Autodesk Inventor part; units mm, degrees
ref_plane "YZ Plane" through (0, 0, 0) normal (1, 0, 0) x (0, 1, 0)
ref_plane "XZ Plane" through (0, 0, 0) normal (0, 1, 0) x (-1, 0, 0)
ref_plane "XY Plane" through (0, 0, 0) normal (0, 0, 1) x (1, 0, 0)
sketch "Sketch2" plane through (0, 0, 0) normal (0, 1, 0) x (-1, 0, 0)
  line L0 (0, 0) -> (88.3, 0)
  line L1 (88.3, 0) -> (88.3, -60)
  line L2 (88.3, -60) -> (0, -60)
  line L3 (0, -60) -> (0, 0)
  line L4 (88.3, -60) -> (68.3, -60)
  line L5 (68.3, 0) -> (68.3, -20)
  line L6 (0, -60) -> (20, -60)
  line L7 (20, 0) -> (20, -20)
  line L8 (20, -20) -> (20, -60)
  line L9 (20, -20) -> (68.3, -20)
  line L10 (68.3, -20) -> (68.3, -60)
  line L11 (68.3, -20) -> (48.3, -20)
  line L12 (48.3, -20) -> (68.3, -40)
  line L13 (20, -20) -> (40, -20)
  line L14 (40, -20) -> (20, -40)
  line L15 (78.3, -60) -> (78.3, -40)
  line L16 (78.3, -40) -> (78.3, -50)
  line L17 (78.3, -40) -> (78.3, -50)
  line L18 (78.3, -40) -> (78.3, -30)
  circle A0 centre (78.3, -30) radius 2.5
  circle A1 centre (78.3, -50) radius 2.5
  line L19 (44.15, -60) -> (44.15, -44.15)
  circle A2 centre (10, -30) radius 2.5
  circle A3 centre (10, -50) radius 2.5
  line L20 (44.15, -20) -> (44.15, -10)
  line L21 (44.15, -10) -> (58.3, -10)
  line L22 (44.15, -10) -> (30, -10)
  circle A4 centre (58.3, -10) radius 2.5
  circle A5 centre (30, -10) radius 2.5
  dimension "d0" = 88.3
  dimension "d1" = 60
  dimension "d2" = 20
  dimension "d3" = 20
  dimension "d4" = 20
  dimension "d5" = 20
  dimension "d6" = 20
  dimension "d7" = 20
  dimension "d9" = 20
  dimension "d10" = 5
  dimension "d11" = 5
  dimension "d12" = 5
  dimension "d13" = 5
extrude "Extrusion1" add sketch "Sketch2" along normal blind 2 contours L0 L7 L8 L2 L3 | L0 L5 L9 L7 | L0 L1 L2 L10 L5 | L9 L14 L8 | L10 L12 L9
sketch "Sketch3" plane through (0, 2, 0) normal (0, 1, 0) x (1, 0, 0)
  line L0 (0, 0) -> (0, 10)
  line L1 (0, 0) -> (0, 60)
  line L2 (0, 10) -> (-10, 10)
  line L3 (-88.2278, 0) -> (-88.3, 9.9997)
  line L4 (-88.3, 60) -> (-88.3, 0)
  line L5 (-88.3, 9.9997) -> (-78.3003, 10.072)
  circle A0 centre (-78.3003, 10.072) radius 2
  circle A1 centre (-10, 10) radius 2
  dimension "d16" = 10
  dimension "d17" = 10
  dimension "d18" = 10
  dimension "d19" = 10
  dimension "d20" = 4
  dimension "d21" = 4
extrude "Extrusion2" cut sketch "Sketch3" against normal blind 2
properties part number "Connect_u2020" material "Aluminum 6061"
Read the model definition and answer for the solid it produces. Units are mm, in the model's axes. A direction names the side the tool comes from. Give positions to 0.01 mm unless a question says otherwise; leave off trailing zeros. Write each loop counter-clockwise with the first axis right and the second up, starting at its lowest first coordinate (ties: lowest second). Pieces come first, ordered by that corner, then holes. Notation, with made-up numbers: (45, 32) - (90, 32) arc R14 ccw to (90, 36) - close; hole circle Ø8 at (27, 13.5). An arc over 180 degrees is marked (long way). Answer in a Markdown table with one row per item. Add a question column.
Item 1: Determine the mould class of faces 1 (the face through (-76.4, 1, -10.7)), 2 (the face through (0, 1, -30)), 3 (the face through (-80.685, 0.986, -50.751)), 4 (the face through (-44, 1, -20)) for opening direction Z: pulls with the +Z half, pulls with the -Z half, needs draft (parallel to the pull), parting line crosses it, or undercut.
Item 2: A tool of negligible diameter and unlimited length cuts with its end or side. For faces 5 (the face through (-44, 2, -16)), 6 (the face through (-30, 1, -30)), from which of +Z, -Z, +X, -X, +Y, -Y can it reach the whole face along a straight path? Write none if from no direction.
Item 3: Section A-A, the plane x = -30 is taken. Write down the section's boundary in (y, z), and give its area (3 significant figures).
Item 4: Section B-B, the plane z = -34 is taken. Write down the section's boundary in (x, y), and give its area (3 significant figures).
Item 5: A flat-ended cylindrical pin translates along its axis: P1, Ø1, axis at x = -43, y = 1, coming from the -Z side. Find the tip coordinate at first contact, or state that the pin passes through.
Item 6: Section D-D, the plane z = -51 is taken. Write down the section's boundary in (x, y), and give its area (3 significant figures).
Item 7: Section C-C, the plane x = -10 is taken. Write down the section's boundary in (y, z), and give its area (3 significant figures).
Item 8: Find the intervals of material crossed by L1, parallel to X at y = 0.65, z = -46.5; L2, parallel to Z at x = -78.3, y = 1.05; L3, parallel to Z at x = -59, y = 0.85, in increasing order.
Recorded:
| question | item | result |
|---|---|---|
| 1 | face 1 | undercut |
| 1 | face 2 | needs draft |
| 1 | face 3 | undercut |
| 1 | face 4 | pulls with the -Z half |
| 2 | face 5 | +Z, -Z, +X, -X, +Y |
| 2 | face 6 | -Z, +Y, -Y |
| 3 | outline | (0, -30) - (2, -30) - (2, -12.5) - (0, -12.5) - close; (0, -7.5) - (2, -7.5) - (2, 0) - (0, 0) - close |
| 3 | area | 50.0 mm2 |
| 4 | outline | (-88.3, 0) - (-62.3, 0) - (-62.3, 2) - (-88.3, 2) - close; (-26, 0) - (0, 0) - (0, 2) - (-26, 2) - close |
| 4 | area | 104 mm2 |
| 5 | P1 | stops at z = -20 |
| 6 | outline | (-88.3, 0) - (-80.59, 0) - (-80.59, 2) - (-88.3, 2) - close; (-76.01, 0) - (-68.3, 0) - (-68.3, 2) - (-76.01, 2) - close; (-20, 0) - (-12.29, 0) - (-12.29, 2) - (-20, 2) - close; (-7.71, 0) - (0, 0) - (0, 2) - (-7.71, 2) - close |
| 6 | area | 61.7 mm2 |
| 7 | outline | (0, -60) - (2, -60) - (2, -52.5) - (0, -52.5) - close; (0, -47.5) - (2, -47.5) - (2, -32.5) - (0, -32.5) - close; (0, -27.5) - (2, -27.5) - (2, -12) - (0, -12) - close; (0, -8) - (2, -8) - (2, 0) - (0, 0) - close |
| 7 | area | 92.0 mm2 |
| 8 | L1 | x = -88.3 to -68.3, -20 to 0 |
| 8 | L2 | z = -60 to -52.5, -47.5 to -32.5, -27.5 to -12.07, -8.07 to 0 |
| 8 | L3 | z = -30.7 to -12.4, -7.6 to 0 |
